Could you check a few things on this model? Use its own coordinates, in mm. Round coordinates to 2 decimals unless told otherwise and drop trailing zeros. Loops run counter-clockwise (first coordinate to the right, second up) from the corner with the lowest first, then second, coordinate; pieces in that order, holes last. Notation, with made-up numbers: (17.25, -19.5) - (49.25, -19.5) arc R16 ccw to (49.25, -11.5) - close; hole circle Ø1 at (81.25, 16.5). An arc over 180 degrees is marked (long way). Use one line per item in the form item = value.
Autodesk Inventor part; units mm, degrees
ref_plane "YZ Plane" through (0, 0, 0) normal (1, 0, 0) x (0, 1, 0)
ref_plane "XZ Plane" through (0, 0, 0) normal (0, 1, 0) x (-1, 0, 0)
ref_plane "XY Plane" through (0, 0, 0) normal (0, 0, 1) x (1, 0, 0)
sketch "Sketch1" plane through (0, 0, 0) normal (0, 0, 1) x (1, 0, 0)
  line L0 (0, -50) -> (-29.4, -50)
  line L1 (-29.4, -50) -> (-29.4, 50)
  line L2 (-29.4, 50) -> (0, 50)
  line L3 (0, 50) -> (0, -50)
  line L4 (0, -13.95) -> (-29.4, -13.95)
  point P0 (0, 0)
  dimension "d0" = 50
  dimension "d1" = 50
  dimension "d2" = 0
extrude "Extrusion1" add sketch "Sketch1" along normal blind 1
sketch "Sketch2" plane through (0, 0, 1) normal (0, 0, 1) x (1, 0, 0)
  circle A0 centre (-8.025, -22.2) radius 1.425
  circle A1 centre (-18.075, -22.2) radius 1.425
  line L0 (-27.4, -19.2) -> (0, -19.2)
  line L1 (-27.4, -19.2) -> (-27.4, -28.5)
  line L2 (-27.4, -28.5) -> (0, -28.5)
  line L3 (0, -19.2) -> (0, -28.5)
  circle A2 centre (-8.025, 22.45) radius 1.2295
  circle A3 centre (-18.075, 22.45) radius 1.2295
  line L4 (-27.4, 19.2) -> (0, 19.2)
  line L5 (0, 19.2) -> (0, 28.5)
  line L6 (0, 28.5) -> (-27.4, 28.5)
  line L7 (-27.4, 19.2) -> (-27.4, 28.5)
  point P0 (0, 0)
hole "Hole1" at (-8.025, -22.2, 1) at (-18.075, -22.2, 1) at (-18.075, 22.45, 1) at (-8.025, 22.45, 1) direction (0, 0, -1) diameter 3 depth 10 countersink diameter 6 countersink angle 90
properties part number "MetalBack" material "Stainless Steel"
1. Please list where these lines run through material, in increasing order: line 1 along Y through (x, z) = (-8, 0.45); line 2 along Y through (x, z) = (-17.5, 0.75); line 3 along X through (y, z) = (20, 0.7).
Solution:
line_1 = -50 to -24.65, -19.75 to 20, 24.9 to 50
line_2 = -50 to -24.89, -19.51 to 19.76, 25.14 to 50
line_3 = -29.4 to -19.21, -16.94 to -9.16, -6.89 to 0
2. If we section it at B-B, the plane z = 0.4: Write out the boundary of the cut face in (x, y) (3 decimals), plus the area to 3 significant figures.
Solution:
outline = (-29.4, -50) - (0, -50) - (0, 50) - (-29.4, 50) - close; hole circle Ø4.8 at (-18.075, -22.2); hole circle Ø4.8 at (-18.075, 22.45); hole circle Ø4.8 at (-8.025, -22.2); hole circle Ø4.8 at (-8.025, 22.45)
area = 2,870 mm^2
3. If we section it at A-A, the plane y = -22.2: Write out the boundary of the cut face in (x, z) (3 decimals), plus the area to 3 significant figures.
Solution:
outline = (-29.4, 0) - (-20.075, 0) - (-21.075, 1) - (-29.4, 1) - close; (-16.075, 0) - (-10.025, 0) - (-11.025, 1) - (-15.075, 1) - close; (-6.025, 0) - (0, 0) - (0, 1) - (-5.025, 1) - close
area = 19.4 mm^2
